Answer from the drawing. Dimensions are ordinates in mm from the lowest x, y and z of the part. Give positions to 0.01 mm unless a question says otherwise; leave off trailing zeros. Write each loop counter-clockwise with the first axis right and the second up, starting at its lowest first coordinate (ties: lowest second). Pieces come first, ordered by that corner, then holes.
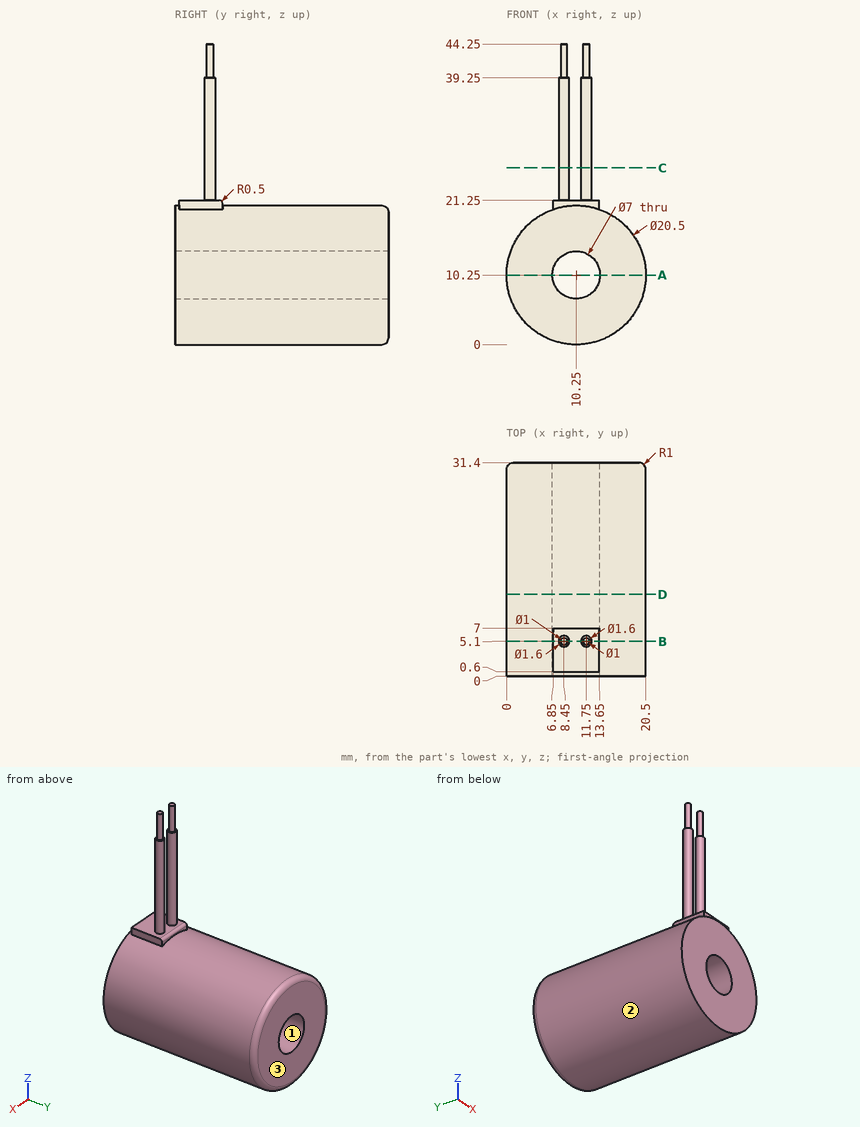
Item 1: Each of these flat-tipped pins is pushed along its axis until it touches: P1, Ø11, axis at x = 10.25, z = 10.25, coming from the +Y side; P2, Ø6, axis at x = 5.5, z = 27, coming from the +Y side; P3, Ø3, axis at x = 6, y = 3.5, coming from the -Z side; P4, Ø2, axis at x = 12.5, y = 26, coming from the +Z side. Where does it stop, or does it pass through?
Conclusion:
P1: stops at y = 31.4
P2: stops at y = 5.9
P3: stops at z = 0.38
P4: stops at z = 20.42
Item 2: Determine the mould class of the marked faces 1, 2 and 3 for opening direction Z: pulls with the +Z half, pulls with the -Z half, needs draft (parallel to the pull), parting line crosses it, or undercut.
Conclusion:
face 1: undercut
face 2: parting line crosses it
face 3: needs draft
Item 3: Consider probe 1 along X at (y, z) = (11.5, 10.25); probe 2 along Z at (x, y) = (10, 10.5); probe 3 along Z at (x, y) = (5.75, 21.5). Determine where each line is inside the solid, lowest interval first.
Conclusion:
probe 1: x = 0 to 6.75, 13.75 to 20.5
probe 2: z = 0 to 6.76, 13.74 to 20.5
probe 3: z = 1.04 to 19.46
Item 4: A cutting plane is placed at C-C, the plane z = 26. Give the vertices of the cut face in (x, y), plus the area to 3 significant figures.
Conclusion:
outline: circle Ø1.6 at (8.45, 5.1); circle Ø1.6 at (11.75, 5.1)
area: 4.02 mm2
Item 5: A cutting plane is placed at B-B, the plane y = 5.1. Give the vertices of the cut face in (x, z), plus the area to 3 significant figures.
Conclusion:
outline: (6.85, 19.92) arc R10.25 ccw (long way) to (13.65, 19.92) - (13.65, 21.25) - (12.55, 21.25) - (12.55, 39.25) - (12.25, 39.25) - (12.25, 44.25) - (11.25, 44.25) - (11.25, 39.25) - (10.95, 39.25) - (10.95, 21.25) - (9.25, 21.25) - (9.25, 39.25) - (8.95, 39.25) - (8.95, 44.25) - (7.95, 44.25) - (7.95, 39.25) - (7.65, 39.25) - (7.65, 21.25) - (6.85, 21.25) - close; hole circle Ø7 at (10.25, 10.25)
area: 366 mm2
Item 6: A cutting plane is placed at A-A, the plane z = 10.25. Give the vertices of the cut face in (x, y).
Conclusion:
outline: (0, 0) - (6.75, 0) - (6.75, 31.4) - (1, 31.4) arc R1 ccw to (0, 30.4) - close; (13.75, 0) - (20.5, 0) - (20.5, 30.4) arc R1 ccw to (19.5, 31.4) - (13.75, 31.4) - close
Item 7: A cutting plane is placed at D-D, the plane y = 12. Give the vertices of the cut face in (x, z).
Conclusion:
outline: circle Ø20.5 at (10.25, 10.25); hole circle Ø7 at (10.25, 10.25)
